from build123d import *

# Parameters (mm, degrees)
ESBO_O1_W                = 101
ESBO_O1_H                = 160
RESSALTO_EXTRUS_O1_DEPTH = 3
ESBO_O2_R                = 1.25
CORTE_EXTRUS_O1_DEPTH    = 140
CHANFRO1_SIZE            = 20
ESBO_O3_W                = 61
ESBO_O3_H                = 3
RESSALTO_EXTRUS_O2_DEPTH = 25
ESBO_O4_R                = 0.5
CORTE_EXTRUS_O2_DEPTH    = 25


with BuildPart() as part:
    # Esboço1 → Ressalto-extrusão1 (new body)
    with BuildSketch(Plane(origin=(0, 0, 0), x_dir=(1, 0, 0), z_dir=(0, 1, 0))):
        with Locations((-30.270258535, -22.046326637)):
            Rectangle(ESBO_O1_W, ESBO_O1_H)
    extrude(amount=RESSALTO_EXTRUS_O1_DEPTH)

    # Esboço2 → Corte-extrusão1 (cut)
    with BuildSketch(Plane(origin=(0, 3, 0), x_dir=(1, 0, 0), z_dir=(0, 1, 0))):
        with Locations((15.229741465, -21.546326637)):
            Circle(ESBO_O2_R)
        with Locations((-75.770258535, -21.546326637)):
            Circle(ESBO_O2_R)
        with Locations((-30.270258535, 25.953673363)):
            Circle(ESBO_O2_R)
        with Locations((-43.770258535, -98.046326637)):
            Circle(ESBO_O2_R)
        with Locations((-16.770258535, -98.046326637)):
            Circle(ESBO_O2_R)
    extrude(amount=-CORTE_EXTRUS_O1_DEPTH, mode=Mode.SUBTRACT)

    # Chanfro1
    chanfro1_edges = [part.edges().sort_by_distance(p)[0] for p in [
        (-80.770258535, 1.5, -57.953673363),
        (20.229741465, 1.5, -57.953673363),
        (20.229741465, 1.5, 102.046326637),
        (-80.770258535, 1.5, 102.046326637),
    ]]
    chamfer(chanfro1_edges, length=CHANFRO1_SIZE)

    # Esboço3 → Ressalto-extrusão2 (add)
    with BuildSketch(Plane.XZ):
        with Locations((-30.270258535, -56.453673363)):
            Rectangle(ESBO_O3_W, ESBO_O3_H)
    extrude(amount=RESSALTO_EXTRUS_O2_DEPTH)

    # Esboço4 → Corte-extrusão2 (cut)
    with BuildSketch(Plane(origin=(0, 0, -57.953673363), x_dir=(-1, 0, 0), z_dir=(0, 0, -1))):
        with Locations((9.770258535, -5.5)):
            Circle(ESBO_O4_R)
        with Locations((50.770258535, -21)):
            Circle(ESBO_O4_R)
        with Locations((9.770258535, -21)):
            Circle(ESBO_O4_R)
        with Locations((50.770258535, -5.5)):
            Circle(ESBO_O4_R)
    extrude(amount=-CORTE_EXTRUS_O2_DEPTH, mode=Mode.SUBTRACT)


solid = part.part
Source: CAD feature listing. Evaluate the final solid. Frame: model axes, mm. A direction names the side the tool comes from. Give positions to 0.01 mm unless a question says otherwise; leave off trailing zeros. Loops run counter-clockwise (first coordinate to the right, second up) from the corner with the lowest first, then second, coordinate; pieces in that order, holes last. Notation, with made-up numbers: (28.25, -8.75) -> (64.25, -8.75) arc R18 cw to (64.25, 22.25) -> close; hole circle Ø11 at (73, 68). An arc over 180 degrees is marked (long way). Use a Markdown table: item, result. Add a question column.
1) Section query A-A, the plane x = -25.5. Return the cut outline in (y, z), then the cut area to 3 significant figures.
2) Section query B-B, the plane z = -22. Return the cut outline in (x, y), then the cut area to 3 significant figures.
3) Reachability of faces 1 (the face through (-80.77, 1, 23)), 2 (the face through (-31, 1, 102.046)), 3 (the face through (-60.77, -12, -56)), 4 (the face through (0.23, -12, -56)), 5 (the face through (-31, -12, -54.954)) from +Z, -Z, +X, -X, +Y, -Y: full face, straight path, thin tool, end or side. Return the list, or none.
4) First-contact query: pin 1 (2 mm diameter, centred on x = -30.27, z = -25.95, fed in from +Y); pin 2 (1.5 mm diameter, centred on x = -55, y = -11.5, fed in from +Z); pin 3 (2.5 mm diameter, centred on y = -17, z = -56.5, fed in from +X); pin 4 (1.5 mm diameter, centred on x = -62, z = 78, fed in from -Y). Flat tips, straight axial feed; report the tip coordinate or a pass-through.
5) Line query: line 1 along Y through (x, z) = (-64, 29.5); line 2 along Z through (x, y) = (-3, -4). Output: solid intervals per line, ascending. Write a range as [from, to].
6) Section query C-C, the plane y = -13.5. Return the cut outline in (x, z).
Numbers:
| question | item | result |
|---|---|---|
| 1 | outline | (-25, -57.95) -> (3, -57.95) -> (3, 102.05) -> (0, 102.05) -> (0, -54.95) -> (-25, -54.95) -> close |
| 1 | area | 555 mm2 |
| 2 | outline | (-80.77, 0) -> (20.23, 0) -> (20.23, 3) -> (-80.77, 3) -> close |
| 2 | area | 303 mm2 |
| 3 | face 1 | +Z, -Z, -X, +Y, -Y |
| 3 | face 2 | +Z, +X, -X, +Y, -Y |
| 3 | face 3 | +Z, -Z, -X, -Y |
| 3 | face 4 | +Z, -Z, +X, -Y |
| 3 | face 5 | +Z, +X, -X, -Y |
| 4 | pin 1 | passes through |
| 4 | pin 2 | stops at z = -54.95 |
| 4 | pin 3 | stops at x = 0.23 |
| 4 | pin 4 | stops at y = 0 |
| 5 | line 1 | y = [0, 3] |
| 5 | line 2 | z = [-57.95, -54.95] |
| 6 | outline | (-60.77, -57.95) -> (0.23, -57.95) -> (0.23, -54.95) -> (-60.77, -54.95) -> close |
